Check sheet for the modelled part. Datum: model origin and axes. Units: mm. Coordinates: 2 decimals unless noted, no trailing zeros. Order: outer loops, then holes, each group sorted by start corner. A loop starts at its lowest first (then second) coordinate and runs counter-clockwise, first axis right, second up.
1. Cross-section at C-C (z = 72.5). Enter the section's corners in (x, y) (3 decimals).
2. Gauge pin test, flat end, axial feed: pin 1 Ø4 at (x, y) = (20, 38) entering from +Z. Record the tip position at first contact, or that the pin passes through.
3. Cross-section at B-B (y = 16). Enter the section's corners in (x, z) (3 decimals), then the cut area to 3 significant figures.
4. Cross-section at D-D (y = 29). Enter the section's corners in (x, z) (3 decimals), then the cut area to 3 significant figures.
5. Thickness scan on line 1 (Z direction, x = 1.5, y = 18); line 2 (X direction, y = 11, z = 95) (3 decimals); line 3 (Y direction, x = 22, z = 181) (3 decimals). Record the ranges inside material, lowest first.
6. Cross-section at A-A (x = 19.5). Enter the section's corners in (y, z) (3 decimals).
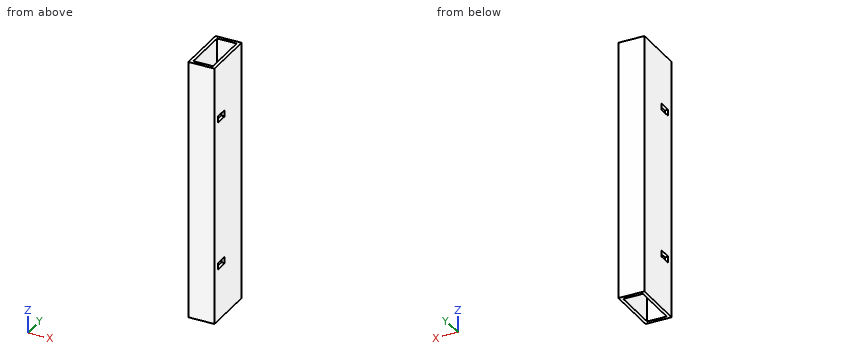
```python
from build123d import *

# Parameters (mm, degrees)
SKETCH1_W           = 25.4
SKETCH1_H           = 50.8
SKETCH1_W_2         = 19.05
SKETCH1_H_2         = 44.45
BOSS_EXTRUDE1_DEPTH = 254
SKETCH2_R           = 6.482173328
CUT_EXTRUDE1_DEPTH  = 254
BOSS_EXTRUDE2_START = -25.4
SKETCH3_R           = 6.482173328
BOSS_EXTRUDE2_DEPTH = 25.4
SKETCH4_W           = 19.05
SKETCH4_H           = 44.45
CUT_EXTRUDE2_DEPTH  = 254
CUT_EXTRUDE3_DEPTH  = 254


with BuildPart() as part:
    # Sketch1 → Boss-Extrude1 (new body)
    with BuildSketch(Plane.XY):
        with Locations((12.7, 25.4)):
            Rectangle(SKETCH1_W, SKETCH1_H)
        with Locations((12.7, 25.4)):
            Rectangle(SKETCH1_W_2, SKETCH1_H_2, mode=Mode.SUBTRACT)
    extrude(amount=BOSS_EXTRUDE1_DEPTH)

    # Sketch2 → Cut-Extrude1 (cut)
    with BuildSketch(Plane(origin=(25.4, 0, 0), x_dir=(0, 0, -1), z_dir=(1, 0, 0))):
        with Locations((-209.55, 12.7)):
            Circle(SKETCH2_R)
        with Locations((-44.45, 12.7)):
            Circle(SKETCH2_R)
    extrude(amount=-CUT_EXTRUDE1_DEPTH, mode=Mode.SUBTRACT)

    # Sketch3 → Boss-Extrude2 (add)
    with BuildSketch(Plane.ZY.offset(BOSS_EXTRUDE2_START)):
        with Locations((209.55, 12.7)):
            Circle(SKETCH3_R)
        with Locations((44.45, 12.7)):
            Circle(SKETCH3_R)
    extrude(amount=BOSS_EXTRUDE2_DEPTH)

    # Sketch4 → Cut-Extrude2 (cut)
    with BuildSketch(Plane.XY.offset(254)):
        with Locations((12.7, 25.4)):
            Rectangle(SKETCH4_W, SKETCH4_H)
    extrude(amount=-CUT_EXTRUDE2_DEPTH, mode=Mode.SUBTRACT)

    # Sketch5 → Cut-Extrude3 (cut)
    with BuildSketch(Plane.ZY):
        Polygon((196.85, 19.05), (196.85, 6.326748406), (203.2, 6.35), (203.2, 19.05), align=None)
        Polygon((57.15, 6.326748406), (50.8, 6.35), (50.8, 19.05), (57.15, 19.05), align=None)
    extrude(amount=-CUT_EXTRUDE3_DEPTH, mode=Mode.SUBTRACT)


solid = part.part
```
Data:
1. outline: (0, 0) - (25.4, 0) - (25.4, 50.8) - (0, 50.8) - close; hole (3.175, 3.175) - (22.225, 3.175) - (22.225, 47.625) - (3.175, 47.625) - close
2. pin 1: passes through
3. outline: (0, 0) - (3.175, 0) - (3.175, 50.8) - (0, 50.8) - close; (0, 57.15) - (3.175, 57.15) - (3.175, 196.85) - (0, 196.85) - close; (0, 203.2) - (3.175, 203.2) - (3.175, 254) - (0, 254) - close; (22.225, 0) - (25.4, 0) - (25.4, 50.8) - (22.225, 50.8) - close; (22.225, 57.15) - (25.4, 57.15) - (25.4, 196.85) - (22.225, 196.85) - close; (22.225, 203.2) - (25.4, 203.2) - (25.4, 254) - (22.225, 254) - close
3. area: 1,530 mm2
4. outline: (0, 0) - (3.175, 0) - (3.175, 254) - (0, 254) - close; (22.225, 0) - (25.4, 0) - (25.4, 254) - (22.225, 254) - close
4. area: 1,610 mm2
5. line 1: z = 0 to 50.8, 57.15 to 196.85, 203.2 to 254
5. line 2: x = 0 to 3.175, 22.225 to 25.4
5. line 3: y = 0 to 3.175, 47.625 to 50.8
6. outline: (0, 0) - (3.175, 0) - (3.175, 254) - (0, 254) - close; (47.625, 0) - (50.8, 0) - (50.8, 254) - (47.625, 254) - close
